Source: CAD feature listing. Evaluate the final solid. Frame: model axes, mm. A direction names the side the tool comes from. Give positions to 0.01 mm unless a question says otherwise; leave off trailing zeros. Order: outer loops, then holes, each group sorted by start corner. A loop starts at its lowest first (then second) coordinate and runs counter-clockwise, first axis right, second up. Notation, with made-up numbers: M 29,-28.5 L 36,-28.5 A30 ccw 36,5.5 Z; hole C 7.5,0.5 d3. An arc over 180 degrees is marked long. Return JSON: item names as keys, results as strings.
from build123d import *

# Parameters (mm, degrees)
Y_KSEKLIK_EKSTR_ZYON1_DEPTH = 15
IZIM2_R                     = 7.5
KES_EKSTR_ZYON1_DEPTH       = 5
RADYUS1_R                   = 26


with BuildPart() as part:
    # Çizim1 → Yükseklik-Ekstrüzyon1 (new body)
    with BuildSketch(Plane.XY):
        with BuildLine():
            Line((-78, 0), (-78, 350))
            ThreePointArc((-78, 350), (224.641702348, 224.641702348), (350, -78))
            Line((350, -78), (0, -78))
            ThreePointArc((0, -78), (-55.154328933, -55.154328933), (-78, 0))
        make_face()
    extrude(amount=Y_KSEKLIK_EKSTR_ZYON1_DEPTH)

    # Çizim2 → Kes-Ekstrüzyon1 (cut)
    with BuildSketch(Plane.XY.offset(15)):
        with Locations((21.213203436, 21.213203436)):
            Circle(IZIM2_R)
        with Locations((7.764571353, -28.977774789)):
            Circle(IZIM2_R)
        with Locations((-28.977774789, 7.764571353)):
            Circle(IZIM2_R)
        with BuildLine():
            Line((26.5, 279), (26.5, 221))
            ThreePointArc((26.5, 221), (0, 194.5), (-26.5, 221))
            Line((-26.5, 221), (-26.5, 279))
            ThreePointArc((-26.5, 279), (0, 305.5), (26.5, 279))
        make_face()
        with BuildLine():
            Line((215.667568262, 178.89801564), (174.655374953, 137.885822331))
            ThreePointArc((174.655374953, 137.885822331), (137.885822331, 137.885822331), (137.885822331, 174.655374953))
            Line((137.885822331, 174.655374953), (178.89801564, 215.667568262))
            ThreePointArc((178.89801564, 215.667568262), (215.667568262, 215.667568262), (215.667568262, 178.89801564))
        make_face()
        with BuildLine():
            Line((221, 26), (279, 26))
            ThreePointArc((279, 26), (305, 0), (279, -26))
            Line((279, -26), (221, -26))
            ThreePointArc((221, -26), (195, 0), (221, 26))
        make_face()
    extrude(amount=-KES_EKSTR_ZYON1_DEPTH, mode=Mode.SUBTRACT)

    # Radyus1
    radyus1_edges = [part.edges().sort_by_distance(p)[0] for p in [
        (-78, 350, 7.5),
        (350, -78, 7.5),
    ]]
    fillet(radyus1_edges, radius=RADYUS1_R)


solid = part.part
1. Set-up query: faces 1 (the face through (195.006, -0.572, 12.535)), 2 (the face through (91, 91, 15)). Return all of +Z, -Z, +X, -X, +Y, -Y with unobstructed straight access to the full face (end or side cutting, diameter ignored); none if empty.
Evaluation:
{"face 1": "+Z", "face 2": "+Z, +X, -X, +Y, -Y"}
2. Section query B-B (x = 295.5). Return loops of the section in (y, z), then the cut area to 3 significant figures.
Evaluation:
{"outline": "M -78,0 L 131,0 L 131,15 L 20.09,15 L 20.09,10 L -20.09,10 L -20.09,15 L -78,15 Z", "area": "2,930 mm^2"}
3. Draft query along Y for faces 3 (the face through (28.14, 18.34, 12.54)), 4 (the face through (164, -78, 7)), 5 (the face through (91, 91, 0)). Return one class per face: pulls with the +Y half, pulls with the -Y half, needs draft (parallel to the pull), parting line crosses it, or undercut.
Evaluation:
{"face 3": "undercut", "face 4": "pulls with the -Y half", "face 5": "needs draft"}
4. First-contact query: pin 1 (16.5 mm diameter, centred on x = -31, y = 5, fed in from +Z); pin 2 (5 mm diameter, centred on x = -20, y = 221, fed in from +Z); pin 3 (5 mm diameter, centred on x = 246.5, z = 4, fed in from +Y); pin 4 (1.5 mm diameter, centred on y = 257.5, z = 10.5, fed in from +X). Flat tips, straight axial feed; report the tip coordinate or a pass-through.
Evaluation:
{"pin 1": "stops at z = 15", "pin 2": "stops at z = 10", "pin 3": "stops at y = 203.96", "pin 4": "stops at x = 188.7"}
5. Ray query, probe 1 along X at (y, z) = (207.5, 10.25); probe 2 along Y at (x, z) = (232, 10.25); probe 3 along X at (y, z) = (141, 13.25). Return the intervals inside material, ascending.
Evaluation:
{"probe 1": "x = -78 to -22.8, 22.8 to 170.73, 221.19 to 240.86", "probe 2": "y = -78 to -26, 26 to 217.1", "probe 3": "x = -78 to 135.23, 177.77 to 289.73"}
6. Section query C-C (y = 187). Return loops of the section in (x, z), then the cut area to 3 significant figures.
Evaluation:
{"outline": "M -78,0 L 258.09,0 L 258.09,15 L 221.16,15 L 221.16,10 L 150.23,10 L 150.23,15 L -78,15 Z", "area": "4,690 mm^2"}
7. Section query D-D (x = 118.5). Return loops of the section in (y, z).
Evaluation:
{"outline": "M -78,0 L 302.23,0 L 302.23,15 L -78,15 Z"}
8. Section query A-A (z = 12.25). Return loops of the section in (x, y).
Evaluation:
{"outline": "M -78,0 A78 ccw 0,-78 L 323.16,-78 A26 ccw 349.1,-50.32 A428 ccw -50.32,349.1 A26 ccw -78,323.16 Z; hole C -28.98,7.76 d15; hole M -26.5,221 A26.5 ccw 26.5,221 L 26.5,279 A26.5 ccw -26.5,279 Z; hole C 7.76,-28.98 d15; hole C 21.21,21.21 d15; hole M 137.89,174.66 A26 ccw 174.66,137.89 L 215.67,178.9 A26 ccw 178.9,215.67 Z; hole M 221,-26 L 279,-26 A26 ccw 279,26 L 221,26 A26 ccw Z"}
